Read the model definition and answer for the solid it produces. Units are mm, in the model's axes. A direction names the side the tool comes from. Coordinates: 2 decimals unless noted, no trailing zeros. Write each loop counter-clockwise with the first axis right and the second up, starting at its lowest first coordinate (ties: lowest second). Pieces come first, ordered by that corner, then holes.
1) The part is cut by section A-A (x = 26). Determine the outline of the cut face in (y, z), then the cut area to 3 significant figures.
2) Which of the six approach directions +Z, -Z, +X, -X, +Y, -Y give full straight-line access (tool end or side, diameter ignored) to faces 4 (the face through (3, 4, 10.811)), 5 (the face through (14, 10, 9.85)), 6 (the face through (33.27, -4.48, -2.16)), 7 (the face through (3.868, -3, 0))?
3) Find the intervals of material crossed by line 1 (Y direction, x = 2.5, z = 0); line 2 (Y direction, x = 22.5, z = -7.75); line 3 (Y direction, x = 14, z = -9.25), in increasing order.
4) The part is cut by section B-B (z = 8). Determine the outline of the cut face in (x, y) (3 decimals).
5) Determine the mould class of faces 1 (the face through (22.554, -0.687, 0.105)), 2 (the face through (3.99, 5.79, -0.09)), 3 (the face through (14, 10, -9.85)) for opening direction Z: +Z half, -Z half, draft (parallel to the pull), parting line (faces both ways), or undercut.
6) Each of these flat-tipped pins is pushed along its axis until it touches: pin 1 Ø12 at (x, z) = (21.5, -6) entering from +Y; pin 2 Ø12 at (y, z) = (9, -2.5) entering from +X; pin 3 Ø2.5 at (y, z) = (4.03, 0) entering from +X; pin 4 Ø2.5 at (x, y) = (14.33, 8.28) entering from +Z. Where does it stop, or does it pass through?
7) The part is cut by section C-C (x = 17.5). Give the number of separate pieces and of enclosed holes in the cut face, then the cut area to 3 significant figures.
from build123d import *

# Parameters (mm, degrees)
SKETCH2_W           = 21.7
SKETCH2_H           = 25.05
SKETCH2_RX          = 9.525
SKETCH2_RY          = 6.35
BOSS_EXTRUDE1_DEPTH = 12.7
SKETCH3_W           = 21.660653916
SKETCH3_H           = 25.05
BOSS_EXTRUDE2_DEPTH = 3
SKETCH5_W           = 18.892037138
SKETCH5_H           = 21.7
BOSS_EXTRUDE3_DEPTH = 2
SKETCH6_W           = 30
SKETCH6_H           = 21.7
BOSS_EXTRUDE4_DEPTH = 4
SKETCH7_W           = 21.7
SKETCH7_H           = 1
SKETCH7_W_2         = 3.175
SKETCH7_H_2         = 3
CUT_EXTRUDE2_DEPTH  = 23
SKETCH7_3_W         = 21.7
SKETCH7_3_H         = 7.272473706
CUT_EXTRUDE3_DEPTH  = 44.803879418
SKETCH11_R          = 1
CUT_EXTRUDE8_DEPTH  = 33.487034031
CUT_EXTRUDE4_REACH  = 47.088
SKETCH9_R           = 1.5
SKETCH10_R          = 2
CUT_EXTRUDE7_DEPTH  = 1
FILLET5_R           = 6.35
FILLET6_R           = 2
FILLET7_R           = 2


with BuildPart() as part:
    # Sketch2 → Boss-Extrude1 (new body)
    with BuildSketch(Plane(origin=(16.497783942, 9.525, 0), x_dir=(0, 0, -1), z_dir=(0.8660254037844379, 0.5000000000000013, 0))):
        Rectangle(SKETCH2_W, SKETCH2_H)
        with Locations(Location((0, 0), (0, 0, 90))):
            Ellipse(SKETCH2_RX, SKETCH2_RY, mode=Mode.SUBTRACT)
    extrude(amount=-BOSS_EXTRUDE1_DEPTH)

    # Sketch3 → Boss-Extrude2 (add)
    with BuildSketch(Plane(origin=(5.499261314, 3.175, 0), x_dir=(0, 0, 1), z_dir=(-0.8660254037844379, -0.5000000000000014, 0))):
        with Locations((-0.019673042, 0)):
            Rectangle(SKETCH3_W, SKETCH3_H)
    extrude(amount=BOSS_EXTRUDE2_DEPTH)

    # Sketch5 → Boss-Extrude3 (add)
    with BuildSketch(Plane(origin=(0, 0, 0), x_dir=(-1, 0, 0), z_dir=(0, 1, 0))):
        with Locations((-13.314265373, 0)):
            Rectangle(SKETCH5_W, SKETCH5_H)
    extrude(amount=-BOSS_EXTRUDE3_DEPTH)

    # Sketch6 → Boss-Extrude4 (add)
    with BuildSketch(Plane.XZ.offset(2)):
        with Locations((18.868246804, 0)):
            Rectangle(SKETCH6_W, SKETCH6_H)
    extrude(amount=BOSS_EXTRUDE4_DEPTH)

    # Sketch7 → Cut-Extrude2 (cut)
    with BuildSketch(Plane(origin=(33.868246804, 0, 0), x_dir=(0, 0, -1), z_dir=(1, 0, 0))):
        with Locations((0, -2.5)):
            Rectangle(SKETCH7_W, SKETCH7_H)
        with Locations((0, -4.5)):
            Rectangle(SKETCH7_W_2, SKETCH7_H_2)
    extrude(amount=-CUT_EXTRUDE2_DEPTH, mode=Mode.SUBTRACT)

    # Sketch7<3> → Cut-Extrude3 (cut, through all)
    with BuildSketch(Plane(origin=(33.868246804, 0, 0), x_dir=(0, 0, -1), z_dir=(1, 0, 0))):
        with Locations((0, -9.636236853)):
            Rectangle(SKETCH7_3_W, SKETCH7_3_H)
    extrude(amount=-CUT_EXTRUDE3_DEPTH, mode=Mode.SUBTRACT)

    # Sketch11 → Cut-Extrude8 (cut, through all)
    with BuildSketch(Plane(origin=(19.672783942, 0.194872981, 0), x_dir=(0, 0, -1), z_dir=(-1, 0, 0))):
        with Locations(Location((0, -3.830865705, 0), (0, 0, 90))):
            Circle(SKETCH11_R)
    extrude(amount=CUT_EXTRUDE8_DEPTH, mode=Mode.SUBTRACT)

    # Sketch9 → Cut-Extrude4 (cut, up to next)
    with BuildSketch(Plane(origin=(0, 0, -10.85), x_dir=(-1, 0, 0), z_dir=(0, 0, -1)), mode=Mode.PRIVATE) as cut_extrude4_sk1:
        with Locations((-14.332720433, 8.275)):
            Circle(SKETCH9_R)
    cut_extrude4_tool1 = extrude(cut_extrude4_sk1.sketch, amount=-CUT_EXTRUDE4_REACH, mode=Mode.PRIVATE) & part.part
    cut_extrude4 = cut_extrude4_tool1.solids().sort_by_distance((14.33272, 8.275, -10.85))[0]
    add(cut_extrude4, mode=Mode.SUBTRACT)

    # Sketch10 → Cut-Extrude7 (cut)
    with BuildSketch(Plane(origin=(0, 0, -10.85), x_dir=(-1, 0, 0), z_dir=(0, 0, -1))):
        with Locations((-14.332720433, 8.275)):
            Circle(SKETCH10_R)
    cut_extrude7 = extrude(amount=-CUT_EXTRUDE7_DEPTH, mode=Mode.SUBTRACT)

    # Mirror1: Cut-Extrude4, Cut-Extrude7 across plane
    add(cut_extrude4.mirror(Plane.XY), mode=Mode.SUBTRACT)
    add(cut_extrude7.mirror(Plane.XY), mode=Mode.SUBTRACT)

    # Fillet5
    fillet5_edges = [part.edges().sort_by_distance(p)[0] for p in [
        (33.868246804, -4.5, 10.85),
        (33.868246804, -4.5, -10.85),
        (22.760283942, -1, -10.85),
        (22.760283942, -1, 10.85),
        (4.736022628, 17.196968182, 10.85),
        (3.436984522, 16.446968182, -10.85),
    ]]
    fillet(fillet5_edges, radius=FILLET5_R)

    # Fillet6
    fillet6_edges = [part.edges().sort_by_distance(p)[0] for p in [
        (33.868246804, -4.5, 1.5875),
        (33.868246804, -4.5, -1.5875),
    ]]
    fillet(fillet6_edges, radius=FILLET6_R)

    # Fillet7
    # the kernel refuses this fillet: 2 mm, written as the material it takes off along each edge
    with BuildSketch(Plane(origin=(22.760283942, 0, 8.429393602), x_dir=(-1, 0, 0), z_dir=(0, 0, -1))) as fillet7_piece_1:
        with BuildLine():
            CenterArc((2, -1.571757441), FILLET7_R, 128.197977663, 51.802022337)
            Line((0, -1.571757441), (-0.04, -1.571757441))
            Line((-0.04, -1.571757441), (-0.04, 0))
            Line((-0.04, 0), (0, 0.04))
            ThreePointArc((0, 0.04), (0.381619343, 0.04), (0.73850346, 0.031435149))
            Line((0.73850346, 0.031435149), (0.763238686, 0))
        make_face()
    extrude(amount=16.858787203, mode=Mode.SUBTRACT)


solid = part.part
Reported:
1. outline: (-6, -10.85) - (-3, -10.85) - (-3, -1.59) - (-6, -1.59) - close; (-6, 1.59) - (-3, 1.59) - (-3, 10.85) - (-6, 10.85) - close
1. area: 55.6 mm2
2. face 4: +Z, -X
2. face 5: +Z
2. face 6: +X, +Y, -Y
2. face 7: +Z, -Z, -X, -Y
3. line 1: y = 2.37 to 3.03, 5.03 to 8.37, 12.44 to 15.91
3. line 2: y = -6 to -3
3. line 3: y = -6 to -3, -2 to 6.81, 9.74 to 13.85
4. outline: (-2.835, 11.611) - (3.868, 0) - (3.868, -6) - (32.817, -6) - (32.817, -3) - (10.868, -3) - (10.868, -2) - (21.709, -2) - (21.709, 0.5) - (10.761, 19.461) - close; hole circle Ø3 at (14.333, 8.275)
5. face 1: draft
5. face 2: undercut
5. face 3: -Z half
6. pin 1: stops at y = 11.25
6. pin 2: stops at x = 20.14
6. pin 3: stops at x = 5.73
6. pin 4: passes through
7. separate pieces: 3
7. enclosed holes: 0
7. area: 189 mm2
